The listing builds one solid part. Answer for the finished solid, in the listing's coordinates (mm). Coordinates: 2 decimals unless noted, no trailing zeros. Order: outer loops, then holes, each group sorted by start corner. A loop starts at its lowest first (then second) coordinate and runs counter-clockwise, first axis right, second up. Notation, with made-up numbers: (-14.5, -39.75) -> (24.5, -39.75) arc R16 cw to (24.5, -11.75) -> close; hole circle Ø11 at (87, -22.75). An arc over 180 degrees is marked (long way). Answer in a Markdown table with one row per item. Add a question column.
```python
from build123d import *

# Parameters (mm, degrees)
SKETCH1_R      = 25
SKETCH1_R_2    = 20
SKETCH1_R_3    = 1.75
SKETCH1_R_4    = 2.5
EXTRUDE1_DEPTH = 0.5


with BuildPart() as part:
    # Sketch1 → Extrude1 (new body)
    with BuildSketch(Plane.XY):
        with BuildLine():
            Line((-60.398675482, 64), (60.398675482, 64))
            ThreePointArc((60.398675482, 64), (0, -88), (-60.398675482, 64))
        make_face()
        Circle(SKETCH1_R, mode=Mode.SUBTRACT)
        with Locations((-35, -54.772255751)):
            Circle(SKETCH1_R_2, mode=Mode.SUBTRACT)
        with Locations((-54.772255751, 35)):
            Circle(SKETCH1_R_2, mode=Mode.SUBTRACT)
        with Locations((54.772255751, 35)):
            Circle(SKETCH1_R_2, mode=Mode.SUBTRACT)
        with Locations((35, -54.772255751)):
            Circle(SKETCH1_R_2, mode=Mode.SUBTRACT)
        with Locations((-75, 10)):
            Circle(SKETCH1_R_3, mode=Mode.SUBTRACT)
        with Locations((0, 56)):
            Circle(SKETCH1_R_3, mode=Mode.SUBTRACT)
        with Locations((0, -74)):
            Circle(SKETCH1_R_3, mode=Mode.SUBTRACT)
        with Locations((75, 10)):
            Circle(SKETCH1_R_3, mode=Mode.SUBTRACT)
        with Locations((-75, -23)):
            Circle(SKETCH1_R_4, mode=Mode.SUBTRACT)
        with Locations((75, -23)):
            Circle(SKETCH1_R_4, mode=Mode.SUBTRACT)
    extrude(amount=EXTRUDE1_DEPTH)


solid = part.part
```
Q1. A cutting plane is placed at C-C (x = 8.5). Determine the outline of the cut face in (y, z), then the cut area to 3 significant figures.
Q2. Straight lines are drawn through the part: line 1 (Y direction, x = 0, z = 0.45); line 2 (X direction, y = 28, z = 0.15); line 3 (X direction, y = 38.5, z = 0.3). For each, find the intervals that lie inside material, in ascending order.
Q3. Determine the mould class of faces 1 (the face through (1, -28, 0.5)), 2 (the face through (2.94, -87.95, 0.25)), 3 (the face through (76.669, 10.526, 0.246)), 4 (the face through (72.5, -22.9, 0.2)) for opening direction X: +X half, -X half, draft (parallel to the pull), parting line (faces both ways), or undercut.
Q4. A cutting plane is placed at A-A (y = 0). Determine the outline of the cut face in (x, z), then the cut area to 3 significant figures.
Q5. A cutting plane is placed at D-D (z = 0.35). State how many separate pieces and enclosed holes the cut face has, then the cut area to 3 significant figures.
Q6. Given pin 1 (2 mm diameter, centred on x = 0, y = 56, fed in from -Z), flat-ended and moving along its own axis, determine where the tip first touches the part or whether it passes through.
Q7. A cutting plane is placed at B-B (x = -46). Determine the outline of the cut face in (y, z), then the cut area to 3 significant figures.
Returned:
| question | item | result |
|---|---|---|
| 1 | outline | (-87.59, 0) -> (-23.51, 0) -> (-23.51, 0.5) -> (-87.59, 0.5) -> close; (23.51, 0) -> (64, 0) -> (64, 0.5) -> (23.51, 0.5) -> close |
| 1 | area | 52.3 mm² |
| 2 | line 1 | y = -88 to -75.75, -72.25 to -25, 25 to 54.25, 57.75 to 64 |
| 2 | line 2 | x = -83.43 to -73.51, -36.04 to 36.04, 73.51 to 83.43 |
| 2 | line 3 | x = -79.13 to -74.46, -35.08 to 35.08, 74.46 to 79.13 |
| 3 | face 1 | draft |
| 3 | face 2 | parting line |
| 3 | face 3 | undercut |
| 3 | face 4 | undercut |
| 4 | outline | (-88, 0) -> (-25, 0) -> (-25, 0.5) -> (-88, 0.5) -> close; (25, 0) -> (88, 0) -> (88, 0.5) -> (25, 0.5) -> close |
| 4 | area | 63.0 mm² |
| 5 | separate pieces | 1 |
| 5 | enclosed holes | 11 |
| 5 | area | 15,300 mm² |
| 6 | pin 1 | passes through |
| 7 | outline | (-75.02, 0) -> (-71.48, 0) -> (-71.48, 0.5) -> (-75.02, 0.5) -> close; (-38.07, 0) -> (17.03, 0) -> (17.03, 0.5) -> (-38.07, 0.5) -> close; (52.97, 0) -> (64, 0) -> (64, 0.5) -> (52.97, 0.5) -> close |
| 7 | area | 34.8 mm² |
